Could you check a few things on this model? Use its own coordinates, in mm. A direction names the side the tool comes from. Give positions to 0.01 mm unless a question says otherwise; leave off trailing zeros. Loops run counter-clockwise (first coordinate to the right, second up) from the corner with the lowest first, then second, coordinate; pieces in that order, holes last.
1. Imagine slicing it at D-D (x = 3.5). List the corners of the cut face in (y, z) for me.
2. Imagine slicing it at A-A (y = -25). Count the separate pieces of the cut face and the enclosed holes in it, plus the area to 3 significant figures.
3. I need wall thicknesses on line 1 along X through (y, z) = (-22, 33); line 2 along Z through (x, y) = (15.5, -25); line 3 along Z through (x, y) = (2, -41). Which ranges of each line are inside material? Lowest first, please.
4. Imagine slicing it at B-B (x = 33). List the corners of the cut face in (y, z) for me, plus the area to 3 significant figures.
5. Thinking about a two-plate mould opening in Y: for faces 1 (the cylindrical face through (36.056, -25.542, 35.785)), 2 (the flat face through (36, -40, 30)), 3 (the flat face through (18, -25, 30)), which applies, +Y half, -Y half, draft (parallel to the pull), parting line (faces both ways), or undercut?
6. For P1, Ø2, axis at y = -37.5, z = 38, coming from the -X side; P2, Ø24, axis at y = -18, z = 38.5, coming from the +X side; P3, Ø6.5, axis at x = 37, z = 20, coming from the -Y side; P4, Ø4, axis at y = -25, z = 38.23, coming from the -X side, each with a flat end and sliding along its axis, tell me the tip position at first contact or that it passes through.
7. For faces 4 (the flat face through (32, -25, 30)), 5 (the flat face through (14, -40, 30)), 6 (the flat face through (36, -10, 30)), which set-ups out of +Z, -Z, +X, -X, +Y, -Y let a thin tool reach every point of the face, with its end or its side?
```python
from build123d import *

# Parameters (mm, degrees)
F0_W     = 50
F0_H     = 50
F1_DEPTH = 10
F2_W     = 8
F2_H     = 30
F3_DEPTH = 40
F5_D     = 5
F6_R     = 0.024142


with BuildPart() as f1:
    # F0 (on Top) → F1 (new body)
    with BuildSketch(Plane.XY):
        with Locations((25, -25)):
            Rectangle(F0_W, F0_H)
    extrude(amount=F1_DEPTH)

    # F2 (on face) → F3 (join)
    with BuildSketch(Plane.XY.offset(10)):
        with Locations((14, -25)):
            Rectangle(F2_W, F2_H)
        with Locations((36, -25)):
            Rectangle(F2_W, F2_H)
    extrude(amount=F3_DEPTH)

    # F5 (through all)
    with Locations(Plane(origin=(10, 0, 0), x_dir=(0, -1, 0), z_dir=(-1, 0, 0))):
        with Locations((25, 38.225368)):
            Hole(F5_D / 2)

    # F6
    f6_edges = [f1.edges().sort_by_distance(p)[0] for p in [
        (40, -25, 50),
    ]]
    fillet(f6_edges, radius=F6_R)


solid = f1.part
```
Derived:
1. outline: (-50, 0) - (0, 0) - (0, 10) - (-50, 10) - close
2. separate pieces: 3
2. enclosed holes: 0
2. area: 1,060 mm2
3. line 1: x = 10 to 18, 32 to 40
3. line 2: z = 0 to 35.73, 40.73 to 50
3. line 3: z = 0 to 10
4. outline: (-50, 0) - (0, 0) - (0, 10) - (-10, 10) - (-10, 50) - (-40, 50) - (-40, 10) - (-50, 10) - close; hole circle Ø5 at (-25, 38.23)
4. area: 1,680 mm2
5. face 1: undercut
5. face 2: -Y half
5. face 3: draft
6. P1: stops at x = 10
6. P2: stops at x = 40
6. P3: stops at y = -40
6. P4: passes through
7. face 4: +Z, +Y, -Y
7. face 5: +Z, +X, -X, -Y
7. face 6: +Z, +X, -X, +Y
